from build123d import *

# Parameters (mm, degrees)
F2_R     = 9.5
F4_W     = 267.021797
F4_H     = 292.826072
F5_DEPTH = 40.8


with BuildPart() as f3:
    # F3: sweep along a path in F0
    with BuildLine(Plane.XY) as f3_path:
        ThreePointArc((0, 100), (29.289322, 29.289322), (100, 0))
    # F2 (on offset) → F3 (sweep)
    with BuildSketch(Plane.YZ.offset(100)):
        Circle(F2_R)
    sweep(path=f3_path.line)

    # F4 (on Front) → F5 (cut)
    with BuildSketch(Plane.XZ):
        with Locations((22.515599, 0.766836)):
            Rectangle(F4_W, F4_H)
    extrude(amount=F5_DEPTH, mode=Mode.SUBTRACT)

    # F6: F3 across face


with BuildPart() as f3_1:
    add(f3.part)
    add(f3.part.mirror(Plane(origin=(80.01217, 0, -7e-06), x_dir=(1, 0, 0), z_dir=(0, -1, 0))))


solid = f3_1.part
The listing builds one solid part. Answer for the finished solid, in the listing's coordinates (mm). Give positions to 0.01 mm unless a question says otherwise; leave off trailing zeros. Loops run counter-clockwise (first coordinate to the right, second up) from the corner with the lowest first, then second, coordinate; pieces in that order, holes last.
Item 1: Find the intervals of material crossed by line 1 along Y through (x, z) = (47.5, 0.5); line 2 along Y through (x, z) = (6.5, -6.75); line 3 along X through (y, z) = (87.5, 6), in increasing order.
Derived:
line 1: y = -26.27 to -3.92, 3.92 to 26.27
line 2: y = -100 to -48.62, 48.62 to 100
line 3: x = -6.64 to 8.21
Item 2: A cutting plane is placed at A-A (z = 6). Give the vertices of the cut face in (x, y), then the cut area to 3 significant figures.
Derived:
outline: (-7.37, -100) - (7.37, -100) arc R92.63 cw to (100, -7.37) - (100, 7.37) arc R92.63 cw to (7.37, 100) - (-7.37, 100) arc R107.37 ccw to (60.92, 0) arc R107.37 ccw to start
area: 4,240 mm2
Item 3: Each of these flat-tipped pins is pushed along its axis until it touches: pin 1 Ø10 at (x, y) = (60, -16.5) entering from -Z; pin 2 Ø3 at (x, z) = (24, -5) entering from +Y; pin 3 Ø1 at (y, z) = (67.5, -5.5) entering from -X; pin 4 Ø6 at (x, y) = (34, 45) entering from -Z. Where does it stop, or does it pass through?
Derived:
pin 1: stops at z = -9.19
pin 2: stops at y = 51.03
pin 3: stops at x = -3.11
pin 4: passes through
Item 4: A cutting plane is placed at B-B (z = -6.75). Give the vertices of the cut face in (x, y), then the cut area to 3 significant figures.
Derived:
outline: (-6.68, -100) - (6.68, -100) arc R93.32 cw to (100, -6.68) - (100, 6.68) arc R93.32 cw to (6.68, 100) - (-6.68, 100) arc R106.68 ccw to (62.83, 0) arc R106.68 ccw to start
area: 3,870 mm2
